Autodesk Inventor part; units mm, degrees
ref_plane "YZ Plane" through (0, 0, 0) normal (1, 0, 0) x (0, 1, 0)
ref_plane "XZ Plane" through (0, 0, 0) normal (0, 1, 0) x (-1, 0, 0)
ref_plane "XY Plane" through (0, 0, 0) normal (0, 0, 1) x (1, 0, 0)
sketch "Sketch1" plane through (0, 0, 0) normal (1, 0, 0) x (0, 1, 0)
  circle A0 centre (0, 0) radius 3.875
  dimension "d0" = 7.75
extrude "Extrusion1" add sketch "Sketch1" along normal blind 21
sketch "Sketch2" plane through (21, 0, 0) normal (1, 0, 0) x (0, 0, -1)
  circle A0 centre (0, 0) radius 2.625
  line L0 (1.9107, -1.8) -> (-1.9107, -1.8)
  line L1 (-2.625, 0) -> (2.625, 0)
  line L2 (1.9107, 1.8) -> (-1.9107, 1.8)
  dimension "d3" = 5.25
  dimension "d4" = 1.8
extrude "Extrusion2" add sketch "Sketch2" along normal blind 7.9 contours L1 A0 L2 | A0 L0 L1
sketch "Sketch3" plane through (28.9, 0, 0) normal (1, 0, 0) x (0, 0, -1)
  circle A0 centre (0, 0) radius 1.15
  dimension "d7" = 2.3
extrude "Extrusion3" cut sketch "Sketch3" against normal through all
properties part number "shaft shooting_3DPrint"
For this review, take the finished solid that the model builds, in its own axes (mm). A direction names the side the tool comes from. Round coordinates to 2 decimals unless told otherwise and drop trailing zeros. Write each loop counter-clockwise with the first axis right and the second up, starting at its lowest first coordinate (ties: lowest second). Pieces come first, ordered by that corner, then holes. Notation, with made-up numbers: (25, 66) - (32, 66) arc R31 cw to (32, 95) - close; hole circle Ø8 at (-16.75, 55.5). An arc over 180 degrees is marked (long way). Put each result on its own line as item: value.
Q1. Insertion check: pin 1 Ø2 at (x, z) = (24.5, 1) entering from -Y; pin 2 Ø4 at (x, y) = (25.5, -0.5) entering from +Z (3 decimals); pin 3 Ø3 at (y, z) = (0, 0) entering from -X; pin 4 Ø1.1 at (x, z) = (26, 0.5) entering from +Y. Each pin has a flat end and moves straight along its axis. Give the tip position at first contact, or say it passes through.
Solved:
pin 1: stops at y = -1.8
pin 2: stops at z = 2.625
pin 3: stops at x = 0
pin 4: stops at y = 1.8
Q2. We need section A-A (y = 0). Give the boundary of the cut face in (x, z) (3 decimals), and give its area (3 significant figures).
Solved:
outline: (0, -3.875) - (21, -3.875) - (21, -2.625) - (28.9, -2.625) - (28.9, -1.15) - (0, -1.15) - close; (0, 1.15) - (28.9, 1.15) - (28.9, 2.625) - (21, 2.625) - (21, 3.875) - (0, 3.875) - close
area: 138 mm2
Q3. We need section C-C (x = 18.75). Give the boundary of the cut face in (y, z) (3 decimals).
Solved:
outline: circle Ø7.75 at (0, 0); hole circle Ø2.3 at (0, 0)
Q4. Machinability: for faces 1 (the face through (24.895, 0.028, -2.625)), 2 (the face through (24.895, -0.028, 2.625)), 3 (the face through (10.353, -0.504, -3.842)), 4 (the face through (21, 3, 0)), which of the approach directions +Z, -Z, +X, -X, +Y, -Y give a long, thin tool a straight path to every point of the face, cutting with its end or side? Answer none if there is none.
Solved:
face 1: -Z, +X
face 2: +Z, +X
face 3: +X, -X
face 4: +X
Q5. Mouldability with a two-part tool opening along Y and no side actions: class faces 5 (the face through (25, 1.8, 0)), 6 (the face through (25, -1.8, 0)), 7 (the face through (14.65, -0.7, 0.91)), 8 (the face through (0, 1, 1)) as released by +Y, released by -Y, zero draft, split by the parting line, or undercut.
Solved:
face 5: released by +Y
face 6: released by -Y
face 7: undercut
face 8: zero draft
Q6. We need section D-D (z = 1.5). Give the boundary of the cut face in (x, y).
Solved:
outline: (0, -3.57) - (21, -3.57) - (21, -1.8) - (28.9, -1.8) - (28.9, 1.8) - (21, 1.8) - (21, 3.57) - (0, 3.57) - close
Q7. We need section B-B (z = 0). Give the boundary of the cut face in (x, y) (3 decimals).
Solved:
outline: (0, -3.875) - (21, -3.875) - (21, -1.8) - (28.9, -1.8) - (28.9, -1.15) - (0, -1.15) - close; (0, 1.15) - (28.9, 1.15) - (28.9, 1.8) - (21, 1.8) - (21, 3.875) - (0, 3.875) - close
Q8. Wall thickness on probe 1 along X at (y, z) = (2, 2.75); probe 2 along Y at (x, z) = (22.5, 0); probe 3 along Y at (x, z) = (27, -0.5): over which ranges is each line inside the solid? List them lowest first.
Solved:
probe 1: x = 0 to 21
probe 2: y = -1.8 to -1.15, 1.15 to 1.8
probe 3: y = -1.8 to -1.04, 1.04 to 1.8
